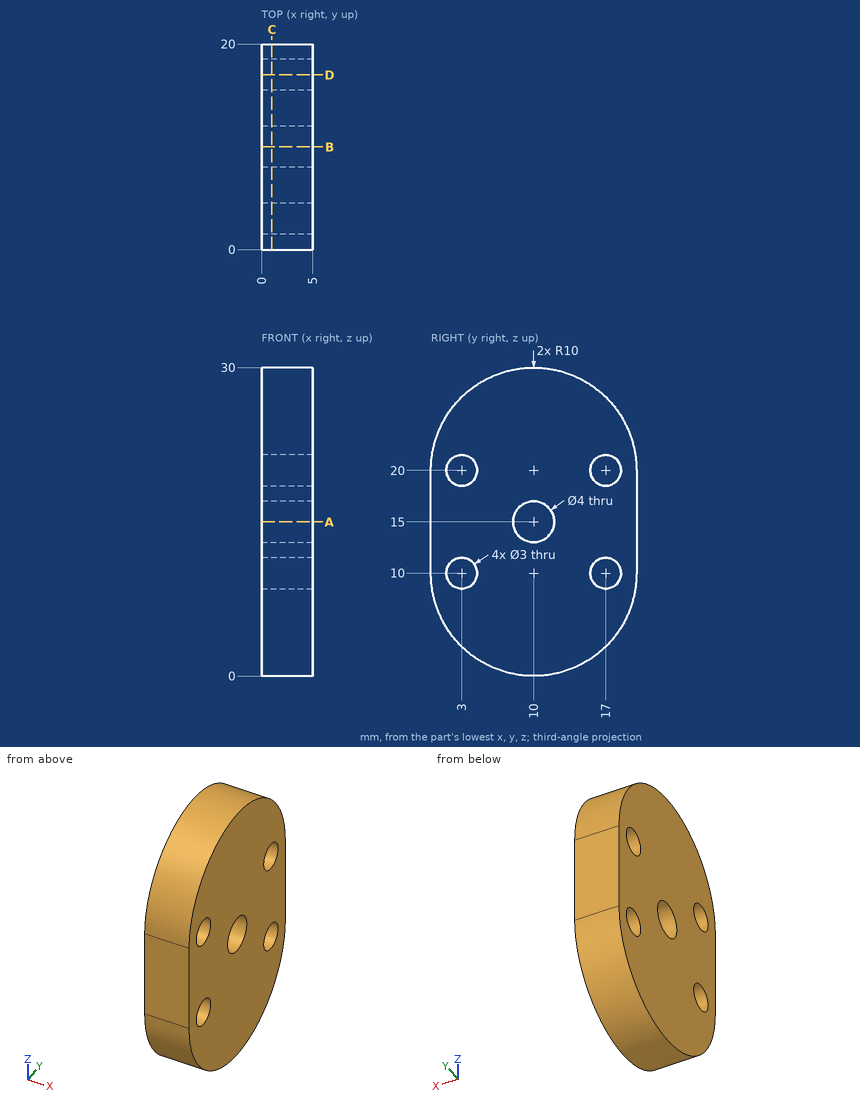
Print and shaded views of the part. All mm, measured from the part's lowest x, y and z. Round coordinates to 2 decimals unless told otherwise and drop trailing zeros. Loops run counter-clockwise (first coordinate to the right, second up) from the corner with the lowest first, then second, coordinate; pieces in that order, holes last. Notation, with made-up numbers: M -17.75,72 L -9.75,72 A20 cw -9.75,108 Z; hole C -6,7.25 d3. An arc over 180 degrees is marked long. One line per question, with ' | ' between items.
1) Band-saw the part on A-A (z = 15). Give the cut face in (x, y).
Solved:
outline: M 0,0 L 5,0 L 5,8 L 0,8 Z; M 0,12 L 5,12 L 5,20 L 0,20 Z
2) Band-saw the part on C-C (x = 1). Give the cut face in (y, z), then the cut area to 3 significant figures.
Solved:
outline: M 0,10 A10 ccw 20,10 L 20,20 A10 ccw 0,20 Z; hole C 3,10 d3; hole C 3,20 d3; hole C 10,15 d4; hole C 17,10 d3; hole C 17,20 d3 | area: 473 mm²
3) Drill centre lines: line 1 along Y through (x, z) = (1.75, 10); line 2 along Z through (x, y) = (1.35, 10); line 3 along Z through (x, y) = (2.4, 3). Where is each one in solid material? Low to high.
Solved:
line 1: y = 0 to 1.5, 4.5 to 15.5, 18.5 to 20 | line 2: z = 0 to 13, 17 to 30 | line 3: z = 2.86 to 8.5, 11.5 to 18.5, 21.5 to 27.14
4) Flat gauge pins, fed straight in: pin 1 (1.5 mm diameter, centred on x = 3, y = 12, fed in from -Z); pin 2 (1.5 mm diameter, centred on x = 1, z = 7.5, fed in from -Y); pin 3 (1 mm diameter, centred on x = 3.5, y = 3, fed in from +Z). Where does each tip first touch, or does it go through?
Solved:
pin 1: stops at z = 0.08 | pin 2: stops at y = 0.15 | pin 3: stops at z = 27.6
5) Band-saw the part on B-B (y = 10). Give the cut face in (x, z).
Solved:
outline: M 0,0 L 5,0 L 5,13 L 0,13 Z; M 0,17 L 5,17 L 5,30 L 0,30 Z
6) Band-saw the part on D-D (y = 17). Give the cut face in (x, z).
Solved:
outline: M 0,2.86 L 5,2.86 L 5,8.5 L 0,8.5 Z; M 0,11.5 L 5,11.5 L 5,18.5 L 0,18.5 Z; M 0,21.5 L 5,21.5 L 5,27.14 L 0,27.14 Z
